Geometry: final body of the model. Coordinates: model frame, mm. A direction names the side the tool comes from. Give positions to 0.01 mm unless a question says otherwise; leave off trailing zeros. Order: outer loops, then holes, each group sorted by start corner. A loop starts at its lowest first (then second) coordinate and runs counter-clockwise, first axis right, second up. Notation, with made-up numbers: (40.25, 9.5) - (70.25, 9.5) arc R24 ccw to (70.25, 30.5) - close; hole circle Ø1 at (52, -40). An arc over 180 degrees is marked (long way). One line per item, written item: value.
Autodesk Inventor part; units mm, degrees
ref_plane "YZ Plane" through (0, 0, 0) normal (1, 0, 0) x (0, 1, 0)
ref_plane "XZ Plane" through (0, 0, 0) normal (0, 1, 0) x (-1, 0, 0)
ref_plane "XY Plane" through (0, 0, 0) normal (0, 0, 1) x (1, 0, 0)
sketch "Skizze1" plane through (0, 0, 0) normal (0, 0, 1) x (1, 0, 0)
  circle A0 centre (0, 0) radius 11
  dimension "d0" = 22
extrude "Extrusion1" add sketch "Skizze1" along normal blind 58
sketch "Skizze2" plane through (0, 0, 58) normal (0, 0, 1) x (1, 0, 0)
  circle A0 centre (0, 0) radius 6.5
  dimension "d3" = 13
extrude "Extrusion2" add sketch "Skizze2" along normal blind 1
sketch "Skizze3" plane through (0, 0, 59) normal (0, 0, 1) x (1, 0, 0)
  circle A0 centre (0, 0) radius 2
  dimension "d6" = 4
extrude "Extrusion3" add sketch "Skizze3" along normal blind 13
sketch "Skizze5" plane through (0, 0, 0) normal (0, 0, -1) x (-1, 0, 0)
  circle A0 centre (0, 0) radius 2
  circle A1 centre (0, 0) radius 3
  dimension "d10" = 6
extrude "Extrusion4" add sketch "Skizze5" along normal blind 2 contours A0 | A1
sketch "Skizze6" plane through (0, 0, -2) normal (0, 0, -1) x (-1, 0, 0)
  circle A0 centre (0, 0) radius 0.75
  dimension "d13" = 1.5
extrude "Extrusion5" add sketch "Skizze6" along normal blind 3
properties part number "Fake Motor"
1) Section A-A, the plane y = 0. Return loops of the section in (x, z).
Answers below:
outline: (-11, 0) - (-3, 0) - (-3, -2) - (-0.75, -2) - (-0.75, -5) - (0.75, -5) - (0.75, -2) - (3, -2) - (3, 0) - (11, 0) - (11, 58) - (6.5, 58) - (6.5, 59) - (2, 59) - (2, 72) - (-2, 72) - (-2, 59) - (-6.5, 59) - (-6.5, 58) - (-11, 58) - close
2) Material intervals for line 1 along Z through (x, y) = (-5.75, -4.25); line 2 along X through (y, z) = (-0.5, 7.5); line 3 along Z through (x, y) = (0.5, -1), sorted ascending.
Answers below:
line 1: 0 to 58
line 2: -10.99 to 10.99
line 3: -2 to 72
3) First-contact query: pin 1 (10 mm diameter, centred on y = 2.5, z = 19, fed in from -X); pin 2 (1.5 mm diameter, centred on x = 5, y = 3, fed in from +Z); pin 3 (2 mm diameter, centred on x = -2, y = -1, fed in from -Z); pin 4 (2 mm diameter, centred on y = 6.5, z = 48.5, fed in from +X). Flat tips, straight axial feed; report the tip coordinate or a pass-through.
Answers below:
pin 1: x = -11
pin 2: z = 59
pin 3: z = -2
pin 4: x = 9.53
4) Section D-D, the plane x = 8.5. Return loops of the section in (y, z).
Answers below:
outline: (-6.98, 0) - (6.98, 0) - (6.98, 58) - (-6.98, 58) - close
5) Section C-C, the plane z = 7. Return loops of the section in (x, y), then the cut area to 3 significant figures.
Answers below:
outline: circle Ø22 at (0, 0)
area: 380 mm^2
6) Set-up query: faces 1 (the face through (-5.158, 3.955, 58.493)), 2 (the face through (0, 0, -5)), 3 (the face through (0.75, -0.03, -3.48)). Return all of +Z, -Z, +X, -X, +Y, -Y with unobstructed straight access to the full face (end or side cutting, diameter ignored); none if empty.
Answers below:
face 1: +Z
face 2: -Z, +X, -X, +Y, -Y
face 3: -Z
